Could you check a few things on this model? Use its own coordinates, in mm. A direction names the side the tool comes from. Round coordinates to 2 decimals unless told otherwise and drop trailing zeros. Order: outer loops, then holes, each group sorted by start corner. A loop starts at its lowest first (then second) coordinate and runs counter-clockwise, first axis right, second up. Notation, with made-up numbers: (70, 33) -> (75, 33) arc R23 ccw to (75, 54) -> close; hole circle Ø9 at (7.5, -3). An arc over 180 degrees is marked (long way). Put each result on its own line as item: value. Start each with the question number.
from build123d import *

# Parameters (mm, degrees)
SKETCH1_W                = 60
SKETCH1_H                = 35
BOSS_EXTRUDE1_DEPTH      = 30
CUT_EXTRUDE1_DEPTH       = 31
F_5_0_5_DIAMETER_HOLE1_D = 5
SKETCH6_W                = 60
SKETCH6_H                = 35
SKETCH6_R                = 17
CUT_EXTRUDE2_DEPTH       = 20


with BuildPart() as part:
    # Sketch1 → Boss-Extrude1 (new body)
    with BuildSketch(Plane(origin=(0, 0, 0), x_dir=(0, 0, -1), z_dir=(1, 0, 0))):
        Rectangle(SKETCH1_W, SKETCH1_H)
    extrude(amount=BOSS_EXTRUDE1_DEPTH)

    # Sketch2 → Cut-Extrude1 (cut, through all)
    with BuildSketch(Plane(origin=(30, 0, 0), x_dir=(0, 0, -1), z_dir=(1, 0, 0))):
        with BuildLine():
            Line((4.5, 2.5), (4.5, -2.5))
            Line((4.5, -2.5), (6.538348415, -2.5))
            ThreePointArc((6.538348415, -2.5), (6.883619648, -1.271133567), (7, 0))
            ThreePointArc((7, 0), (6.883619648, 1.271133567), (6.538348415, 2.5))
            Line((6.538348415, 2.5), (4.5, 2.5))
        make_face()
        with BuildLine():
            Line((6.538348415, -2.5), (4.5, -2.5))
            Line((4.5, -2.5), (4.5, 2.5))
            Line((4.5, 2.5), (6.538348415, 2.5))
            ThreePointArc((6.538348415, 2.5), (-7, 0), (6.538348415, -2.5))
        make_face()
        with BuildLine():
            ThreePointArc((7, 0), (6.883619648, -1.271133567), (6.538348415, -2.5))
            Line((6.538348415, -2.5), (9.5, -2.5))
            Line((9.5, -2.5), (9.5, 2.5))
            Line((9.5, 2.5), (6.538348415, 2.5))
            ThreePointArc((6.538348415, 2.5), (6.883619648, 1.271133567), (7, 0))
        make_face()
    extrude(amount=-CUT_EXTRUDE1_DEPTH, mode=Mode.SUBTRACT)

    # Ø5.0 (5) Diameter Hole1 (through all)
    with Locations(Plane.ZY):
        with Locations((-23, 10.5), (-23, -10.5)):
            f_5_0_5_diameter_hole1 = Hole(F_5_0_5_DIAMETER_HOLE1_D / 2)

    # Mirror1: Ø5.0 (5) Diameter Hole1 across plane
    add(f_5_0_5_diameter_hole1.mirror(Plane.XY), mode=Mode.SUBTRACT)

    # Sketch6 → Cut-Extrude2 (cut)
    with BuildSketch(Plane.ZY):
        Rectangle(SKETCH6_W, SKETCH6_H)
        Circle(SKETCH6_R, mode=Mode.SUBTRACT)
    extrude(amount=-CUT_EXTRUDE2_DEPTH, mode=Mode.SUBTRACT)


solid = part.part
1. I need wall thicknesses on L1, parallel to Y at x = 26, z = 23; L2, parallel to Y at x = 14.25, z = 0; L3, parallel to Y at x = 28.25, z = -7.5. Which ranges of each line are inside material? Lowest first, please.
2. For pin 1 Ø6 at (x, y) = (16.5, -2) entering from +Z; pin 2 Ø2 at (x, z) = (19.5, 3.5) entering from +Y; pin 3 Ø3 at (y, z) = (-10.5, 23) entering from +X; pin 4 Ø6 at (y, z) = (12.5, -20.5) entering from -X, each with a flat end and sliding along its axis, tell me the tip position at first contact or that it passes through.
3. If we section it at C-C, the plane y = 1: Please give me the cut outline in (x, z).
4. Which directions (+Z, -Z, +X, -X, +Y, -Y) give clear straight access to the entire face, cutting with the end or side of a thin tool? Please do faces 1 (the face through (9.86, 14.334, 9.139)), 2 (the face through (25, 17.5, 0)), 3 (the face through (15, -2.5, -8)).
5. If we section it at B-B, the plane x = 25.75: Please give me the cut outline in (y, z).
6. Thinking about a two-plate mould opening in Z: for faces 4 (the face through (15, 2.5, -8)), 5 (the face through (25, 9, 21)), 6 (the face through (30, 4, 7)), 7 (the face through (25, 0, 30)), which applies, +Z half, -Z half, draft (parallel to the pull), parting line (faces both ways), or undercut?
7. If we section it at A-A, the plane z = 0: Please give me the cut outline in (x, y).
8. If we section it at D-D, the plane z = 23: Please give me the cut outline in (x, y), then the cut area to 3 significant figures.
Results below:
1. L1: -17.5 to -13, -8 to 8, 13 to 17.5
1. L2: -17 to -7, 7 to 17
1. L3: -17.5 to -2.5, 2.5 to 17.5
2. pin 1: z = 17
2. pin 2: y = 17.5
2. pin 3: through
2. pin 4: x = 20
3. outline: (0, -16.97) -> (20, -16.97) -> (20, -30) -> (30, -30) -> (30, -9.5) -> (0, -9.5) -> close; (0, 6.93) -> (30, 6.93) -> (30, 30) -> (20, 30) -> (20, 16.97) -> (0, 16.97) -> close
4. face 1: -X
4. face 2: +Z, -Z, +X, -X, +Y
4. face 3: +X, -X
5. outline: (-17.5, -30) -> (17.5, -30) -> (17.5, 30) -> (-17.5, 30) -> close; hole circle Ø5 at (-10.5, -23); hole circle Ø5 at (-10.5, 23); hole (-2.5, -9.5) -> (2.5, -9.5) -> (2.5, -6.54) arc R7 ccw (long way) to (-2.5, -6.54) -> close; hole circle Ø5 at (10.5, -23); hole circle Ø5 at (10.5, 23)
6. face 4: undercut
6. face 5: undercut
6. face 6: draft
6. face 7: +Z half
7. outline: (0, -17) -> (20, -17) -> (20, -17.5) -> (30, -17.5) -> (30, -7) -> (0, -7) -> close; (0, 7) -> (30, 7) -> (30, 17.5) -> (20, 17.5) -> (20, 17) -> (0, 17) -> close
8. outline: (20, -17.5) -> (30, -17.5) -> (30, -13) -> (20, -13) -> close; (20, -8) -> (30, -8) -> (30, 8) -> (20, 8) -> close; (20, 13) -> (30, 13) -> (30, 17.5) -> (20, 17.5) -> close
8. area: 250 mm2
